Geometry: final body of the model. Coordinates: model frame, mm. A direction names the side the tool comes from. Give positions to 0.01 mm unless a question says otherwise; leave off trailing zeros. Loops run counter-clockwise (first coordinate to the right, second up) from the corner with the lowest first, then second, coordinate; pieces in that order, holes last. Notation, with made-up numbers: M 15,49 L 57,49 A21 cw 57,55 Z; hole C 13.25,45 d3. An arc over 180 degrees is marked long. Put each result on its own line as item: value.
```python
from build123d import *

# Parameters (mm, degrees)
SKETCH1_W             = 76.2
SKETCH1_H             = 50.8
BOSS_EXTRUDE1_DEPTH   = 6.35
SKETCH2_R             = 3.175
CUT_EXTRUDE1_DEPTH    = 64.816710194
SKETCH3_R             = 4.7625
CUT_EXTRUDE2_DEPTH    = 64.816710194
F_8_CLEARANCE_HOLE1_D = 4.4958
SKETCH6_R             = 3.429
CUT_EXTRUDE3_DEPTH    = 4.572
SKETCH7_R             = 1.5875
CUT_EXTRUDE4_DEPTH    = 47.228697797


with BuildPart() as part:
    # Sketch1 → Boss-Extrude1 (new body)
    with BuildSketch(Plane(origin=(0, 0, 0), x_dir=(1, 0, 0), z_dir=(0, 1, 0))):
        Rectangle(SKETCH1_W, SKETCH1_H)
    extrude(amount=BOSS_EXTRUDE1_DEPTH)

    # Sketch2 → Cut-Extrude1 (cut, through all)
    with BuildSketch(Plane.XY.offset(25.4)):
        with Locations((-25.4, 0)):
            Circle(SKETCH2_R)
        with Locations((25.4, 0)):
            Circle(SKETCH2_R)
    extrude(amount=-CUT_EXTRUDE1_DEPTH, mode=Mode.SUBTRACT)

    # Sketch3 → Cut-Extrude2 (cut, through all)
    with BuildSketch(Plane.XY.offset(25.4)):
        with Locations((-9.525, 0)):
            Circle(SKETCH3_R)
        with Locations((9.525, 0)):
            Circle(SKETCH3_R)
    extrude(amount=-CUT_EXTRUDE2_DEPTH, mode=Mode.SUBTRACT)

    # #8 Clearance Hole1 (through all)
    with Locations(Plane(origin=(0, 6.35, 0), x_dir=(1, 0, 0), z_dir=(0, 1, 0))):
        with Locations((-33.3375, 12.7), (-33.3375, -12.7), (-18.288, -12.7), (0, -12.7), (18.288, -12.7), (33.3375, -12.7), (33.3375, 12.7), (18.288, 12.7), (0, 12.7), (-18.288, 12.7)):
            Hole(F_8_CLEARANCE_HOLE1_D / 2)

    # Sketch6 → Cut-Extrude3 (cut)
    with BuildSketch(Plane(origin=(0, 6.35, 0), x_dir=(1, 0, 0), z_dir=(0, 1, 0))):
        with Locations(Location((-33.3375, 12.7, 0), (0, 0, 270))):
            Circle(SKETCH6_R)
        with Locations(Location((-18.288, 12.7, 0), (0, 0, 270))):
            Circle(SKETCH6_R)
        with Locations(Location((0, 12.7, 0), (0, 0, 270))):
            Circle(SKETCH6_R)
        with Locations(Location((18.288, 12.7, 0), (0, 0, 270))):
            Circle(SKETCH6_R)
        with Locations(Location((33.3375, 12.7, 0), (0, 0, 270))):
            Circle(SKETCH6_R)
        with Locations(Location((33.3375, -12.7, 0), (0, 0, 270))):
            Circle(SKETCH6_R)
        with Locations(Location((18.288, -12.7, 0), (0, 0, 270))):
            Circle(SKETCH6_R)
        with Locations(Location((0, -12.7, 0), (0, 0, 270))):
            Circle(SKETCH6_R)
        with Locations(Location((-18.288, -12.7, 0), (0, 0, 270))):
            Circle(SKETCH6_R)
        with Locations(Location((-33.3375, -12.7, 0), (0, 0, 270))):
            Circle(SKETCH6_R)
    extrude(amount=-CUT_EXTRUDE3_DEPTH, mode=Mode.SUBTRACT)

    # Sketch7 → Cut-Extrude4 (cut, through all)
    with BuildSketch(Plane(origin=(0, 6.35, 0), x_dir=(1, 0, 0), z_dir=(0, 1, 0))):
        with Locations(Location((0, 0, 0), (0, 0, 270))):
            Circle(SKETCH7_R)
    extrude(amount=-CUT_EXTRUDE4_DEPTH, mode=Mode.SUBTRACT)


solid = part.part
```
Item 1: Set-up query: faces 5 (the flat face through (19, 1.778, 15)), 6 (the flat face through (18, 0, 0)). Return all of +Z, -Z, +X, -X, +Y, -Y with unobstructed straight access to the full face (end or side cutting, diameter ignored); none if empty.
Output values:
face 5: +Y
face 6: +Z, -Z, +X, -X, -Y
Item 2: Section B-B on y = 5.5. Count the separate pieces of the cut face and the enclosed holes in it, then the cut area to 3 significant figures.
Output values:
separate pieces: 1
enclosed holes: 11
area: 3,490 mm²
Item 3: Line query: probe 1 along X at (y, z) = (4.95, 12.7); probe 2 along Z at (x, y) = (18, 3.5); probe 3 along Z at (x, y) = (15.5, 4.5). Output: solid intervals per line, ascending. Write a range as [from, to].
Output values:
probe 1: [-38.1, -36.77], [-29.91, -21.72], [-14.86, -3.43], [3.43, 14.86], [21.72, 29.91], [36.77, 38.1]
probe 2: [-25.4, -16.12], [-9.28, 9.28], [16.12, 25.4]
probe 3: [-25.4, -14.7], [-10.7, 10.7], [14.7, 25.4]
Item 4: Mould query, pull axis Z, two halves, no side actions, for faces 1 (the flat face through (18, 1.778, -10)), 2 (the flat face through (-1, 4, -25.4)), 3 (the flat face through (38.1, 3, 0)), 4 (the cylindrical face through (0.29, 0.88, -14.93)). Classes: pulls with the +Z half, pulls with the -Z half, needs draft (parallel to the pull), parting line crosses it, or undercut.
Output values:
face 1: undercut
face 2: pulls with the -Z half
face 3: needs draft
face 4: undercut
Item 5: Pin query (flat end, axial travel): pin 1 Ø3.5 at (x, z) = (32.5, -13) entering from +Y. Return the tip coordinate at first contact, or that it passes through.
Output values:
pin 1: y = 1.78
Item 6: Section D-D on x = -25.4. Output: boundary loops of the cut face in (y, z) (3 decimals), then the cut area to 3 significant figures.
Output values:
outline: M 3.175,-25.4 L 6.35,-25.4 L 6.35,25.4 L 3.175,25.4 Z
area: 161 mm²
